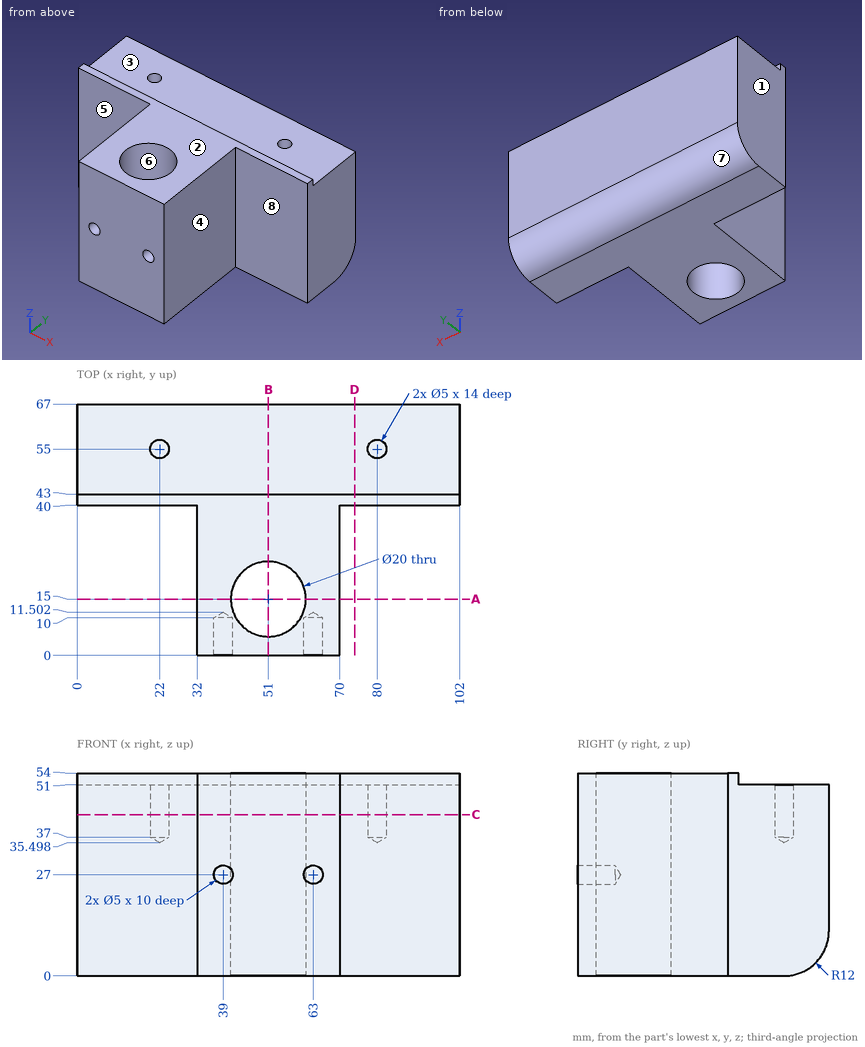
Geometry: see drawing. Coordinates: mm, zero at the bounding-box minimum. A direction names the side the tool comes from. Give positions to 0.01 mm unless a question says otherwise; leave off trailing zeros. Order: outer loops, then holes, each group sorted by start corner. A loop starts at its lowest first (then second) coordinate and runs counter-clockwise, first axis right, second up. Notation, with made-up numbers: (47.5, 49) -> (102.5, 49) arc R25 cw to (102.5, 68) -> close; hole circle Ø11 at (-39.75, 73). An arc over 180 degrees is marked (long way). Write each question's results on one line, items separated by ' | '.
1) Draft query along Y for the marked faces 6, 7 and 8. Return one class per face: released by +Y, released by -Y, zero draft, split by the parting line, or undercut.
Geometry says:
face 6: undercut | face 7: released by +Y | face 8: released by -Y
2) First-contact query: pin 1 Ø4.5 at (x, y) = (22, 55) entering from +Z; pin 2 Ø2 at (y, z) = (15, 18) entering from +X; pin 3 Ø6 at (x, y) = (80, 55) entering from +Z. Flat tips, straight axial feed; report the tip coordinate or a pass-through.
Geometry says:
pin 1: stops at z = 36.85 | pin 2: stops at x = 70 | pin 3: stops at z = 51
3) Cut plane B-B (x = 51). Output: boundary loops of the cut face in (y, z).
Geometry says:
outline: (0, 0) -> (5, 0) -> (5, 54) -> (0, 54) -> close; (25, 0) -> (55, 0) arc R12 ccw to (67, 12) -> (67, 51) -> (43, 51) -> (43, 54) -> (25, 54) -> close
4) Cut plane A-A (y = 15). Output: boundary loops of the cut face in (x, z).
Geometry says:
outline: (32, 0) -> (41, 0) -> (41, 54) -> (32, 54) -> close; (61, 0) -> (70, 0) -> (70, 54) -> (61, 54) -> close
5) Line query: line 1 along X through (y, z) = (55, 41); line 2 along Z through (x, y) = (39, 3); line 3 along X through (y, z) = (6.75, 27). Output: solid intervals per line, ascending.
Geometry says:
line 1: x = 0 to 19.5, 24.5 to 77.5, 82.5 to 102 | line 2: z = 0 to 24.5, 29.5 to 54 | line 3: x = 32 to 36.5, 41.5 to 45.35, 56.65 to 60.5, 65.5 to 70
6) Cut plane D-D (x = 74). Output: boundary loops of the cut face in (y, z), and give its area (3 significant figures).
Geometry says:
outline: (40, 0) -> (55, 0) arc R12 ccw to (67, 12) -> (67, 51) -> (43, 51) -> (43, 54) -> (40, 54) -> close | area: 1,360 mm²
7) Cut plane C-C (z = 43). Output: boundary loops of the cut face in (x, y), and give its area (3 significant figures).
Geometry says:
outline: (0, 40) -> (32, 40) -> (32, 0) -> (70, 0) -> (70, 40) -> (102, 40) -> (102, 67) -> (0, 67) -> close; hole circle Ø5 at (22, 55); hole circle Ø20 at (51, 15); hole circle Ø5 at (80, 55) | area: 3,920 mm²
8) Set-up query: the marked faces 1, 2, 3, 4 and 5. Return all of +Z, -Z, +X, -X, +Y, -Y with unobstructed straight access to the full face (end or side cutting, diameter ignored); none if empty.
Geometry says:
face 1: +Z, -Z, -X, +Y, -Y | face 2: +Z, +X, -X, +Y, -Y | face 3: +Z, +X, -X, +Y | face 4: +Z, -Z, +X, -Y | face 5: +Z, -Z, -X, -Y
